Autodesk Inventor part; units mm, degrees
ref_plane "YZ Plane" through (0, 0, 0) normal (1, 0, 0) x (0, 1, 0)
ref_plane "XZ Plane" through (0, 0, 0) normal (0, 1, 0) x (-1, 0, 0)
ref_plane "XY Plane" through (0, 0, 0) normal (0, 0, 1) x (1, 0, 0)
sketch "Sketch1" plane through (0, 0, 0) normal (0, 0, 1) x (1, 0, 0)
  point P0 (0, 0)
sketch "Sketch2" plane through (0, 0, 0) normal (0, 0, 1) x (1, 0, 0)
  point P0 (0, 0)
sketch "Sketch3" plane through (0, 0, 0) normal (0, 0, 1) x (1, 0, 0)
  line L0 (0, 0) -> (11.1, 0)
  line L1 (11.1, 0) -> (11.1, 13.9)
  line L2 (11.1, 13.9) -> (0, 13.9)
  line L3 (0, 13.9) -> (0, 0)
  line L4 (-1, -1) -> (12.1, -1)
  line L5 (12.1, -1) -> (12.1, 14.9)
  line L6 (12.1, 14.9) -> (-1, 14.9)
  line L7 (-1, 14.9) -> (-1, -1)
  dimension "d0" = 13.9
  dimension "d1" = 11.1
  dimension "d7" = 1
extrude "Extrusion1" add sketch "Sketch3" along normal blind 2
sketch "Sketch5" plane through (0, 0, 0) normal (0, 0, -1) x (-1, 0, 0)
  line L0 (-12.1, 14.9) -> (1, 14.9)
  line L1 (-12.1, -1) -> (-12.1, 14.9)
  line L2 (1, 14.9) -> (1, -1)
  line L3 (1, -1) -> (-12.1, -1)
  line L4 (2.3, 16.2) -> (-13.4, 16.2)
  line L5 (-13.4, 16.2) -> (-13.4, -2.3)
  line L6 (-13.4, -2.3) -> (2.3, -2.3)
  line L7 (2.3, -2.3) -> (2.3, 16.2)
  point P0 (0, 0)
  dimension "d8" = 1.3
extrude "Extrusion2" add sketch "Sketch5" along normal blind 2 contours L0 L2 L3 L1 | L7 L6 L5 L4
sketch "Sketch6" plane through (0, 0, 0) normal (0, 0, 1) x (1, 0, 0)
  circle A0 centre (2.45, 2.45) radius 1.45
  line L0 (0, 0) -> (0, 13.9)
  line L1 (11.1, 0) -> (0, 0)
  dimension "d11" = 2.9
  dimension "d12" = 2.45
  dimension "d13" = 2.45
extrude "Extrusion3" add sketch "Sketch6" along normal blind 2
sketch "Sketch7" plane through (0, 0, 0) normal (0, 0, 1) x (1, 0, 0)
  line L0 (5.1, 3.5) -> (11.1, 3.5)
  line L1 (11.1, 3.5) -> (11.1, 6.5)
  line L2 (11.1, 6.5) -> (5.1, 6.5)
  line L3 (5.1, 6.5) -> (5.1, 3.5)
  line L4 (0, 0) -> (0, 13.9)
  line L5 (11.1, 0) -> (0, 0)
  line L6 (11.1, 13.9) -> (11.1, 0)
  dimension "d16" = 3
  dimension "d17" = 6
  dimension "d22" = 3.5
  dimension "d23" = 0
extrude "Extrusion4" cut sketch "Sketch7" against normal blind 2
fillet "Fillet1" radius 2 4 edges at (13.4, 16.2, -1) (-2.3, 16.2, -1) (13.4, -2.3, -1) (-2.3, -2.3, -1)
chamfer "Chamfer1" distance 1 angle 45 8 edges at (5.55, 16.2, -2) (12.8142, 15.6142, -2) (13.4, 6.95, -2) (12.8142, -1.7142, -2) (5.55, -2.3, -2) (-1.7142, -1.7142, -2) (-2.3, 6.95, -2) (-1.7142, 15.6142, -2)
equation "\"d13\" = d12"
properties part number "VL53L0X_cover"
Work out the finished part from the listing and answer in its coordinate system (mm). A direction names the side the tool comes from. Coordinates: 2 decimals unless noted, no trailing zeros. Order: outer loops, then holes, each group sorted by start corner. A loop starts at its lowest first (then second) coordinate and runs counter-clockwise, first axis right, second up. Notation, with made-up numbers: (4, -37) - (15, -37) arc R14 cw to (15, -32) - close; hole circle Ø8 at (4, 85.5). An arc over 180 degrees is marked (long way). Put each result on its own line as item: value. Start each with the question number.
1) Find section A-A (z = 0.7). Give the vertices of the cut face in (x, y), plus the area to 3 significant figures.
2) For faces 1 (the flat face through (8, 3.5, -1)), 2 (the conical face through (12.4, 15.18, -1.6)), 3 (the flat face through (5.6, -2.3, -0.5)), 4 (the flat face through (6, 14.9, 1)), 5 (the cylindrical face through (2.136, 3.866, 0.986)), determine the directions among +Z, -Z, +X, -X, +Y, -Y from which every point of the face is accessible in a straight line to the end or side of a thin tool.
3) Find section C-C (z = -0.7). Give the vertices of the cut face in (x, y), plus the area to 3 significant figures.
4) For a pull along Y with two mould halves and no side action, classify faces 6 (the cylindrical face through (-1.73, 15.6, -0.51)), 7 (the flat face through (12.9, 6.8, -1.5)), 8 (the cylindrical face through (-1.7, -1.73, -0.51)), 9 (the flat face through (5, 0, 1)) as released by +Y, released by -Y, zero draft, split by the parting line, or undercut.
5) Flat-ended cylindrical pins translate along their axes: pin 1 (1.6 mm diameter, centred on y = 9.5, z = 1, fed in from +X); pin 2 (1.6 mm diameter, centred on x = 6, z = 1.5, fed in from -Y); pin 3 (1 mm diameter, centred on y = 3, z = 1.5, fed in from -X). Find the tip coordinate at first contact, or state that the pin passes through.
6) Find section D-D (y = 2.45). Give the vertices of the cut face in (x, z).
7) Find the intervals of material crossed by line 1 (Y direction, x = 8.5, z = 1.5); line 2 (X direction, y = 11, z = 0.1); line 3 (Y direction, x = 2.75, z = 1.75), in increasing order. Write a range as from..to.
8) Find section B-B (x = 10.75). Give the vertices of the cut face in (y, z), plus the area to 3 significant figures.
Results list:
1. outline: (-1, -1) - (12.1, -1) - (12.1, 14.9) - (-1, 14.9) - close; circle Ø2.9 at (2.45, 2.45); hole (0, 0) - (11.1, 0) - (11.1, 13.9) - (0, 13.9) - close
1. area: 60.6 mm^2
2. face 1: +Z, -Z
2. face 2: -Z, +X, +Y
2. face 3: +Z, -Z, +X, -X, -Y
2. face 4: +Z, +X, -X, +Y
2. face 5: +Z
3. outline: (-2.3, -0.3) arc R2 ccw to (-0.3, -2.3) - (11.4, -2.3) arc R2 ccw to (13.4, -0.3) - (13.4, 14.2) arc R2 ccw to (11.4, 16.2) - (-0.3, 16.2) arc R2 ccw to (-2.3, 14.2) - close; hole (5.1, 3.5) - (11.1, 3.5) - (11.1, 6.5) - (5.1, 6.5) - close
3. area: 269 mm^2
4. face 6: released by +Y
4. face 7: zero draft
4. face 8: released by -Y
4. face 9: undercut
5. pin 1: stops at x = 12.1
5. pin 2: stops at y = -1
5. pin 3: stops at x = -1
6. outline: (-2.3, -1) - (-1.3, -2) - (12.4, -2) - (13.4, -1) - (13.4, 0) - (12.1, 0) - (12.1, 2) - (11.1, 2) - (11.1, 0) - (3.9, 0) - (3.9, 2) - (1, 2) - (1, 0) - (0, 0) - (0, 2) - (-1, 2) - (-1, 0) - (-2.3, 0) - close
7. line 1: y = -1..0, 13.9..14.9
7. line 2: x = -1..0, 11.1..12.1
7. line 3: y = -1..0, 1.03..3.87, 13.9..14.9
8. outline: (-2.3, -1) - (-1.3, -2) - (3.5, -2) - (3.5, 0) - (0, 0) - (0, 2) - (-1, 2) - (-1, 0) - (-2.3, 0) - close; (6.5, -2) - (15.2, -2) - (16.2, -1) - (16.2, 0) - (14.9, 0) - (14.9, 2) - (13.9, 2) - (13.9, 0) - (6.5, 0) - close
8. area: 34.0 mm^2
